from build123d import *

# Parameters (mm, degrees)
BOSS_EXTRUDE1_DEPTH = 6.35
CUT_EXTRUDE1_DEPTH  = 6.35


with BuildPart() as part:
    # Sketch1 → Boss-Extrude1 (new body)
    with BuildSketch(Plane.XY):
        Polygon((-101.6, 19.05), (-101.6, 25.4), (-76.2, 25.4), (-76.2, 19.05), (76.2, 19.05), (76.2, 25.4), (101.6, 25.4), (101.6, 19.05), (139.7, 19.05), (139.7, -19.05), (-139.7, -19.05), (-139.7, 19.05), align=None)
    extrude(amount=BOSS_EXTRUDE1_DEPTH)

    # Sketch2 → Cut-Extrude1 (cut)
    with BuildSketch(Plane.XY.offset(6.35)):
        Polygon((-134.8232, 19.05), (-134.8232, 12.065), (-136.525, 12.065), (-136.525, 8.89), (-134.8232, 8.89), (-134.8232, 6.35), (-131.8768, 6.35), (-131.8768, 8.89), (-130.175, 8.89), (-130.175, 12.065), (-131.8768, 12.065), (-131.8768, 19.05), align=None)
        Polygon((131.8768, 12.065), (131.8768, 19.05), (134.8232, 19.05), (134.8232, 12.065), (136.525, 12.065), (136.525, 8.89), (134.8232, 8.89), (134.8232, 6.35), (131.8768, 6.35), (131.8768, 8.89), (130.175, 8.89), (130.175, 12.065), align=None)
    extrude(amount=-CUT_EXTRUDE1_DEPTH, mode=Mode.SUBTRACT)


solid = part.part
CAD build for the part. Positions are in the model's coordinates, mm. A direction names the side the tool comes from. Give positions to 0.01 mm unless a question says otherwise; leave off trailing zeros. Order: outer loops, then holes, each group sorted by start corner. A loop starts at its lowest first (then second) coordinate and runs counter-clockwise, first axis right, second up. Notation, with made-up numbers: (41, 30) -> (89, 30) arc R6 ccw to (89, 35) -> close; hole circle Ø8 at (-11.75, -24.75). An arc over 180 degrees is marked (long way). Return JSON: item names as keys, results as strings.
Q1. Drill centre lines: line 1 (X direction, y = 19, z = 5); line 2 (Y direction, x = 108, z = 6); line 3 (X direction, y = 20, z = 2.75). Where is each one in solid material? Low to high.
Working result:
{"line 1": "-139.7 to -134.82, -131.88 to 131.88, 134.82 to 139.7", "line 2": "-19.05 to 19.05", "line 3": "-101.6 to -76.2, 76.2 to 101.6"}
Q2. Saw through at A-A (x = -113). Write the cut outline in (y, z), then the cut area to 3 significant figures.
Working result:
{"outline": "(-19.05, 0) -> (19.05, 0) -> (19.05, 6.35) -> (-19.05, 6.35) -> close", "area": "242 mm²"}
Q3. Mould opens along X. For faces 6 (the face through (89, 25.4, 3)), 7 (the face through (101.6, 22, 3)), 8 (the face through (-134.823, 16, 3)), 9 (the face through (-101.6, 22, 3)) say: pulls with the +X half, pulls with the -X half, needs draft (parallel to the pull), parting line crosses it, or undercut.
Working result:
{"face 6": "needs draft", "face 7": "pulls with the +X half", "face 8": "undercut", "face 9": "pulls with the -X half"}
Q4. Which spindle directions (+Z, -Z, +X, -X, +Y, -Y) get a long thin tool onto all of the face, cutting with end or side? Do faces 1 (the face through (2, -19.05, 3)), 2 (the face through (-76.2, 22, 3)), 3 (the face through (117, 19.05, 3)), 4 (the face through (-139.7, 0, 3)), 5 (the face through (-117, 19.05, 3)). Say none if no direction does.
Working result:
{"face 1": "+Z, -Z, +X, -X, -Y", "face 2": "+Z, -Z, +Y", "face 3": "+Z, -Z, +X, +Y", "face 4": "+Z, -Z, -X, +Y, -Y", "face 5": "+Z, -Z, -X, +Y"}
Q5. Flat gauge pin, fed straight in: pin 1 (3 mm diameter, centred on x = 52.5, z = 0.5, fed in from +Y). Where does the tip first touch, or does it go through?
Working result:
{"pin 1": "y = 19.05"}
